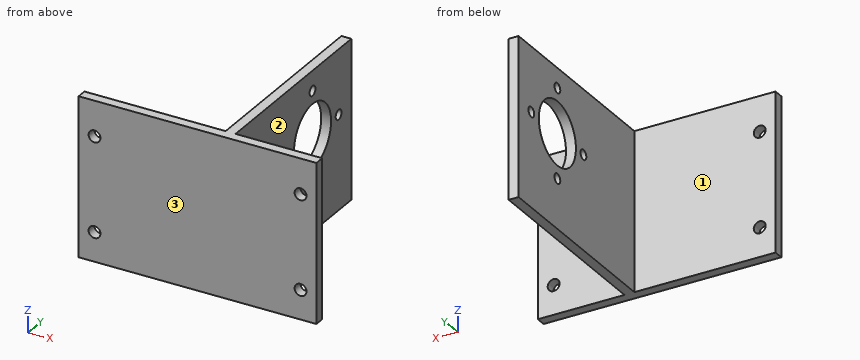
```python
from build123d import *

# Parameters (mm, degrees)
SKETCH1_W               = 120
SKETCH1_H               = 80
SKETCH1_R               = 3
BOSS_EXTRUDE1_DEPTH     = 5
SKETCH2_W               = 5
SKETCH2_H               = 80
BOSS_EXTRUDE2_DEPTH     = 100
CUT_EXTRUDE1_DEPTH      = 136.790509609
CUT_EXTRUDE1_DEPTH_BACK = 136.790509609
SKETCH3_R               = 16
SKETCH3_R_2             = 2.5


with BuildPart() as part:
    # Sketch1 → Boss-Extrude1 (new body)
    with BuildSketch(Plane(origin=(0, 0, 0), x_dir=(1, 0, 0), z_dir=(0, 1, 0))):
        Rectangle(SKETCH1_W, SKETCH1_H)
        with Locations(Location((-52, 25.25, 0), (0, 0, 270))):
            Circle(SKETCH1_R, mode=Mode.SUBTRACT)
        with Locations(Location((-52, -22.25, 0), (0, 0, 270))):
            Circle(SKETCH1_R, mode=Mode.SUBTRACT)
        with Locations(Location((52, -22.25, 0), (0, 0, 270))):
            Circle(SKETCH1_R, mode=Mode.SUBTRACT)
        with Locations(Location((52, 25.25, 0), (0, 0, 270))):
            Circle(SKETCH1_R, mode=Mode.SUBTRACT)
    extrude(amount=BOSS_EXTRUDE1_DEPTH)

    # Sketch2 → Boss-Extrude2 (add)
    with BuildSketch(Plane(origin=(0, 5, 0), x_dir=(1, 0, 0), z_dir=(0, 1, 0))):
        with Locations((13.75, 0)):
            Rectangle(SKETCH2_W, SKETCH2_H)
    extrude(amount=BOSS_EXTRUDE2_DEPTH)

    # Sketch3 → Cut-Extrude1 (cut, two sides: drawn at the far end of the back side and taken through both)
    with BuildSketch(Plane(origin=(16.25, 0, 0), x_dir=(0, 0, -1), z_dir=(1, 0, 0)).offset(-CUT_EXTRUDE1_DEPTH_BACK)):
        with Locations((-7.473800103, 71.5)):
            Circle(SKETCH3_R)
        with Locations((-29.973800103, 71.5)):
            Circle(SKETCH3_R_2)
        with Locations((15.026199897, 71.5)):
            Circle(SKETCH3_R_2)
        with Locations((-7.473800103, 49)):
            Circle(SKETCH3_R_2)
        with Locations((-7.473800103, 94)):
            Circle(SKETCH3_R_2)
    extrude(amount=CUT_EXTRUDE1_DEPTH + CUT_EXTRUDE1_DEPTH_BACK, mode=Mode.SUBTRACT)


solid = part.part
```
Work out the finished part from the listing and answer in its coordinate system (mm). Face numbers are marked on the shaded views. A direction names the side the tool comes from. Round coordinates to 2 decimals unless told otherwise and drop trailing zeros. Loops run counter-clockwise (first coordinate to the right, second up) from the corner with the lowest first, then second, coordinate; pieces in that order, holes last.
(1) The part is cut by section A-A, the plane z = -25.25. Give the vertices of the cut face in (x, y), and give its area (3 significant figures).
Computed values:
outline: (-60, 0) - (-55, 0) - (-55, 5) - (-60, 5) - close; (-49, 0) - (49, 0) - (49, 5) - (16.25, 5) - (16.25, 105) - (11.25, 105) - (11.25, 5) - (-49, 5) - close; (55, 0) - (60, 0) - (60, 5) - (55, 5) - close
area: 1,040 mm2
(2) The part is cut by section D-D, the plane y = 94. Give the vertices of the cut face in (x, z), and give its area (3 significant figures).
Computed values:
outline: (11.25, -40) - (16.25, -40) - (16.25, 4.97) - (11.25, 4.97) - close; (11.25, 9.97) - (16.25, 9.97) - (16.25, 40) - (11.25, 40) - close
area: 375 mm2
(3) Find the intervals of material crossed by L1, parallel to X at y = 3.35, z = -25.25; L2, parallel to Y at x = -28.5, z = -5; L3, parallel to X at y = 54, z = 2, in increasing order.
Computed values:
L1: x = -60 to -55, -49 to 49, 55 to 60
L2: y = 0 to 5
L3: x = 11.25 to 16.25
(4) Each of these flat-tipped pins is pushed along its axis until it touches: P1, Ø10, axis at y = 91, z = 26.5, coming from the +X side; P2, Ø5, axis at x = 52, z = 22.25, coming from the -Y side; P3, Ø10, axis at y = 13, z = 31.5, coming from the -X side; P4, Ø21.5, axis at x = -10.5, z = -11, coming from the +Y side. Where does it stop, or does it pass through?
Computed values:
P1: stops at x = 16.25
P2: passes through
P3: stops at x = 11.25
P4: stops at y = 5
(5) For the marked faces 1, 2 and 3, determine the directions among +Z, -Z, +X, -X, +Y, -Y from which every point of the face is accessible in a straight line to the end or side of a thin tool.
Computed values:
face 1: +Z, -Z, -X, +Y
face 2: +Z, -Z, +X, +Y
face 3: +Z, -Z, +X, -X, -Y
(6) The part is cut by section B-B, the plane x = 52. Give the vertices of the cut face in (y, z), and give its area (3 significant figures).
Computed values:
outline: (0, -40) - (5, -40) - (5, -28.25) - (0, -28.25) - close; (0, -22.25) - (5, -22.25) - (5, 19.25) - (0, 19.25) - close; (0, 25.25) - (5, 25.25) - (5, 40) - (0, 40) - close
area: 340 mm2
(7) The part is cut by section C-C, the plane y = 71.5. Give the vertices of the cut face in (x, z), and give its area (3 significant figures).
Computed values:
outline: (11.25, -40) - (16.25, -40) - (16.25, -17.53) - (11.25, -17.53) - close; (11.25, -12.53) - (16.25, -12.53) - (16.25, -8.53) - (11.25, -8.53) - close; (11.25, 23.47) - (16.25, 23.47) - (16.25, 27.47) - (11.25, 27.47) - close; (11.25, 32.47) - (16.25, 32.47) - (16.25, 40) - (11.25, 40) - close
area: 190 mm2
